Check sheet for the modelled part. Datum: model origin and axes. Units: mm. A direction names the side the tool comes from. Give positions to 0.01 mm unless a question says otherwise; leave off trailing zeros. Order: outer loops, then holes, each group sorted by start corner. A loop starts at its lowest first (then second) coordinate and runs counter-clockwise, first axis right, second up.
Item 1: Sectioned sample at D-D on x = 60. Record the boundary of the cut face in (y, z), and give its area (3 significant figures).
Item 2: Material ranges on line 1 along X through (y, z) = (21, -3); line 2 along X through (y, z) = (23, -21); line 3 along Y through (x, z) = (55, -29.5), recorded low to high.
Item 3: Sectioned sample at A-A on y = 45. Record the boundary of the cut face in (x, z), and give its area (3 significant figures).
Item 4: Sectioned sample at C-C on y = 39. Record the boundary of the cut face in (x, z), and give its area (3 significant figures).
Item 5: Release check for a two-part mould opening along X. For faces 3 (the cylindrical face through (65.58, 47.996, -15.238)), 4 (the flat face through (106.496, 24.178, -15.238)), 5 (the flat face through (65.2, 48.2, -32)) record: released by +X, released by -X, zero draft, split by the parting line, or undercut.
Item 6: Access from +Z, -Z, +X, -X, +Y, -Y to the whole of each face (thin tool, end or side, straight path). Record for faces 1 (the cylindrical face through (64.392, 49.996, -15.238)), 2 (the flat face through (104.897, 22.939, -15.238)).
Item 7: Gauge pin test, flat ends, axial feed: P1, Ø1, axis at x = 52.5, z = -26.5, coming from the +Y side; P2, Ø6, axis at x = 80.5, z = -13, coming from the +Y side; P3, Ø1.5, axis at x = 56.5, z = -3, coming from the -Y side; P4, Ø10, axis at x = 58, y = 39.5, coming from the +Z side. Record the tip position at first contact, or that the pin passes through.
Item 8: Sectioned sample at B-B on z = -13. Record the boundary of the cut face in (x, y).
from build123d import *

# Parameters (mm, degrees)
BOSS_EXTRUDE1_DEPTH      = 2
BOSS_EXTRUDE1_DEPTH_BACK = 32


with BuildPart() as part:
    # Sketch2 → Boss-Extrude1 (new, two sides: drawn at the far end of the back side and taken through both)
    with BuildSketch(Plane.XY.offset(-BOSS_EXTRUDE1_DEPTH_BACK)):
        with BuildLine():
            Line((102.5, 31.332843133), (110.605952255, 16.81955568))
            ThreePointArc((110.605952255, 16.81955568), (110.22051471, 15.458880149), (108.859839179, 15.844317694))
            Line((108.859839179, 15.844317694), (100.821862298, 30.235898765))
            ThreePointArc((100.821862298, 30.235898765), (65, 48), (29.178137702, 30.235898765))
            Line((29.178137702, 30.235898765), (21.140160821, 15.844317694))
            ThreePointArc((21.140160821, 15.844317694), (19.77948529, 15.458880149), (19.394047745, 16.81955568))
            Line((19.394047745, 16.81955568), (27.5, 31.332843133))
            ThreePointArc((27.5, 31.332843133), (65, 50), (102.5, 31.332843133))
        make_face()
    extrude(amount=BOSS_EXTRUDE1_DEPTH + BOSS_EXTRUDE1_DEPTH_BACK)


solid = part.part
Report:
1. outline: (47.72, -32) - (49.73, -32) - (49.73, 2) - (47.72, 2) - close
1. area: 68.4 mm2
2. line 1: x = 21.73 to 24.02, 105.98 to 108.27
2. line 2: x = 22.85 to 25.14, 104.86 to 107.15
2. line 3: y = 46.87 to 48.92
3. outline: (43.9, -32) - (48.84, -32) - (48.84, 2) - (43.9, 2) - close; (81.16, -32) - (86.1, -32) - (86.1, 2) - (81.16, 2) - close
3. area: 336 mm2
4. outline: (34.78, -32) - (38, -32) - (38, 2) - (34.78, 2) - close; (92, -32) - (95.22, -32) - (95.22, 2) - (92, 2) - close
4. area: 219 mm2
5. face 3: undercut
5. face 4: released by +X
5. face 5: zero draft
6. face 1: +Z, -Z, +Y
6. face 2: +Z, -Z, -Y
7. P1: stops at y = 48.44
7. P2: stops at y = 48.31
7. P3: stops at y = 47.04
7. P4: passes through
8. outline: (19.39, 16.82) arc R1 ccw to (21.14, 15.84) - (29.18, 30.24) arc R45 cw to (100.82, 30.24) - (108.86, 15.84) arc R1 ccw to (110.61, 16.82) - (102.5, 31.33) arc R47 ccw to (27.5, 31.33) - close
